```python
from build123d import *

# Parameters (mm, degrees)
SKETCH1_W           = 30
SKETCH1_H           = 50
BOSS_EXTRUDE1_DEPTH = 1
SKETCH2_W           = 1
SKETCH2_H           = 50
BOSS_EXTRUDE2_DEPTH = 30
FILLET2_R           = 2
FILLET3_R           = 0.5


with BuildPart() as part:
    # Sketch1 → Boss-Extrude1 (new body)
    with BuildSketch(Plane.XY):
        with Locations((15, 25)):
            Rectangle(SKETCH1_W, SKETCH1_H)
    extrude(amount=BOSS_EXTRUDE1_DEPTH)

    # Sketch2 → Boss-Extrude2 (add)
    with BuildSketch(Plane.XY.offset(1)):
        with Locations((0.5, 25)):
            Rectangle(SKETCH2_W, SKETCH2_H)
        with Locations((7.6, 25)):
            Rectangle(SKETCH2_W, SKETCH2_H)
    extrude(amount=BOSS_EXTRUDE2_DEPTH)

    # Fillet2
    fillet2_edges = [part.edges().sort_by_distance(p)[0] for p in [
        (1, 25, 1),
        (7.1, 25, 1),
        (8.1, 25, 1),
    ]]
    fillet(fillet2_edges, radius=FILLET2_R)

    # Fillet3
    fillet3_edges = [part.edges().sort_by_distance(p)[0] for p in [
        (1, 25, 31),
        (7.1, 25, 31),
    ]]
    fillet(fillet3_edges, radius=FILLET3_R)


solid = part.part
```
Verification items for the finished model (mm, model axes). A direction names the side the tool comes from. Coordinates: 2 decimals unless noted, no trailing zeros. Loops run counter-clockwise (first coordinate to the right, second up) from the corner with the lowest first, then second, coordinate; pieces in that order, holes last. Notation, with made-up numbers: (-38, 56) - (19, 56) arc R20 cw to (19, 87) - close; hole circle Ø5 at (-14.5, 56.25). An arc over 180 degrees is marked (long way). Return JSON: item names as keys, results as strings.
1. Thickness scan on L1, parallel to X at y = 18.5, z = 12; L2, parallel to Z at x = 24, y = 46; L3, parallel to Z at x = 5.75, y = 17. Record the ranges inside material, lowest first.
Established:
{"L1": "x = 0 to 1, 7.1 to 8.1", "L2": "z = 0 to 1", "L3": "z = 0 to 1.11"}
2. Section check A-A, the plane z = 6.5. Record the boundary of the cut face in (x, y), then the cut area to 3 significant figures.
Established:
{"outline": "(0, 0) - (1, 0) - (1, 50) - (0, 50) - close; (7.1, 0) - (8.1, 0) - (8.1, 50) - (7.1, 50) - close", "area": "100 mm2"}
3. Tool access check on faces 1 (the flat face through (20, 25, 1)), 2 (the flat face through (30, 24.7, 0.5)), 3 (the cylindrical face through (6.53, 25.35, 1.6)). Record the directions out of +Z, -Z, +X, -X, +Y, -Y that give a thin tool (end or side, any length) a straight path to the whole face; none if there is none.
Established:
{"face 1": "+Z, +X, +Y, -Y", "face 2": "+Z, -Z, +X, +Y, -Y", "face 3": "+Z, +Y, -Y"}
4. Section check C-C, the plane x = 15. Record the boundary of the cut face in (y, z).
Established:
{"outline": "(0, 0) - (50, 0) - (50, 1) - (0, 1) - close"}
5. Section check D-D, the plane x = 6.5. Record the boundary of the cut face in (y, z).
Established:
{"outline": "(0, 0) - (50, 0) - (50, 1.57) - (0, 1.57) - close"}
6. Section check B-B, the plane y = 19. Record the boundary of the cut face in (x, z), then the cut area to 3 significant figures.
Established:
{"outline": "(0, 0) - (30, 0) - (30, 1) - (10.1, 1) arc R2 cw to (8.1, 3) - (8.1, 31) - (7.6, 31) arc R0.5 ccw to (7.1, 30.5) - (7.1, 3) arc R2 cw to (5.1, 1) - (3, 1) arc R2 cw to (1, 3) - (1, 30.5) arc R0.5 ccw to (0.5, 31) - (0, 31) - close", "area": "92.5 mm2"}
7. Mould release check, pull along X, two halves, no side actions. Record for faces 4 (the cylindrical face through (8.7, 25.35, 1.57)), 5 (the flat face through (4, 25, 1)), 6 (the cylindrical face through (1.6, 25.35, 1.57)), 7 (the flat face through (15, 25, 0)): +X half, -X half, draft (parallel to the pull), parting line (faces both ways), or undercut.
Established:
{"face 4": "+X half", "face 5": "undercut", "face 6": "undercut", "face 7": "draft"}
8. Go/stop test with flat-tipped pins: pin 1 (12 mm diameter, centred on x = 15, z = 8.5, fed in from +Y); pin 2 (1.7 mm diameter, centred on x = 4, y = 26.5, fed in from +Z); pin 3 (8.5 mm diameter, centred on y = 25.5, z = 13.5, fed in from +X); pin 4 (12 mm diameter, centred on x = 15.5, y = 12.5, fed in from +Z). Record where each tip stops, or that it passes through.
Established:
{"pin 1": "passes through", "pin 2": "stops at z = 1", "pin 3": "stops at x = 8.1", "pin 4": "stops at z = 1.09"}
